Check sheet for the modelled part. Datum: model origin and axes. Units: mm. Face numbers are marked on the shaded views. A direction names the side the tool comes from. Coordinates: 2 decimals unless noted, no trailing zeros. Loops run counter-clockwise (first coordinate to the right, second up) from the corner with the lowest first, then second, coordinate; pieces in that order, holes last. Notation, with made-up numbers: (-26, -19.5) - (-22, -19.5) arc R14 ccw to (-22, 2.5) - close; hole circle Ø7 at (-33, 31.25). An arc over 180 degrees is marked (long way). Use a Markdown table: item, result. Add a question column.
1) Sectioned sample at D-D, the plane y = 11.5. Enter the section's corners in (x, z), then the cut area to 3 significant figures.
2) Sectioned sample at B-B, the plane x = 58. Enter the section's corners in (y, z), then the cut area to 3 significant figures.
3) Tool access check on the marked faces 4, 5, 6, 7 and 8. Record the directions out of +Z, -Z, +X, -X, +Y, -Y that give a thin tool (end or side, any length) a straight path to the whole face; none if there is none.
4) Thickness scan on line 1 (Y direction, x = 20, z = 9); line 2 (Z direction, x = 51.5, y = 18); line 3 (X direction, y = 25, z = -4.5). Record the ranges inside material, lowest first.
5) Go/stop test with flat-tipped pins: P1, Ø24, axis at x = 21.5, z = -36, coming from the -Y side; P2, Ø17.5, axis at x = 29.5, y = 60, coming from the -Z side; P3, Ø11, axis at x = 74, z = -43, coming from the -Y side; P4, Ø10, axis at y = 57.5, z = -71, coming from the -X side. Record where each tip stops, or that it passes through.
6) Sectioned sample at C-C, the plane x = 9. Enter the section's corners in (y, z).
7) Sectioned sample at A-A, the plane y = 40. Enter the section's corners in (x, z), then the cut area to 3 significant figures.
8) Draft check along Z on the marked faces 1, 2 and 3. Enter one of: pulls with the +Z half, pulls with the -Z half, needs draft (parallel to the pull), parting line crosses it, or undercut.
from build123d import *

# Parameters (mm, degrees)
BOSS_EXTRUDE1_DEPTH = 12
CUT_EXTRUDE1_REACH  = 115.772
SKETCH2_R           = 5
BOSS_EXTRUDE2_DEPTH = 10
SKETCH8_R           = 20
BOSS_EXTRUDE3_DEPTH = 30
CUT_EXTRUDE2_REACH  = 132.48
SKETCH9_R           = 12.5
BOSS_EXTRUDE4_DEPTH = 5


with BuildPart() as part:
    # Sketch1 → Boss-Extrude1 (new body)
    with BuildSketch(Plane.XY):
        with BuildLine():
            Line((20, 0), (80, 0))
            Line((80, 0), (80, 80))
            Line((80, 80), (20, 80))
            ThreePointArc((20, 80), (5.857864376, 74.142135624), (0, 60))
            Line((0, 60), (0, 20))
            ThreePointArc((0, 20), (5.857864376, 5.857864376), (20, 0))
        make_face()
    extrude(amount=BOSS_EXTRUDE1_DEPTH)

    # Sketch2 → Cut-Extrude1 (cut, up to next)
    with BuildSketch(Plane.XY.offset(12), mode=Mode.PRIVATE) as cut_extrude1_sk1:
        with Locations((20, 65)):
            Circle(SKETCH2_R)
    cut_extrude1_tool1 = extrude(cut_extrude1_sk1.sketch, amount=-CUT_EXTRUDE1_REACH, mode=Mode.PRIVATE) & part.part
    # Sketch2 → Cut-Extrude1 (cut, up to next)
    with BuildSketch(Plane.XY.offset(12), mode=Mode.PRIVATE) as cut_extrude1_sk2:
        with Locations((20, 15)):
            Circle(SKETCH2_R)
    cut_extrude1_tool2 = extrude(cut_extrude1_sk2.sketch, amount=-CUT_EXTRUDE1_REACH, mode=Mode.PRIVATE) & part.part
    add(cut_extrude1_tool1.solids().sort_by_distance((20, 65, 12))[0], mode=Mode.SUBTRACT)
    add(cut_extrude1_tool2.solids().sort_by_distance((20, 15, 12))[0], mode=Mode.SUBTRACT)

    # Sketch5 → Boss-Extrude2 (add)
    with BuildSketch(Plane(origin=(80, 0, 0), x_dir=(0, 0, -1), z_dir=(1, 0, 0))):
        with BuildLine():
            Line((10, 70), (65, 70))
            ThreePointArc((65, 70), (95, 40), (65, 10))
            Line((65, 10), (10, 10))
            ThreePointArc((10, 10), (2.928932188, 7.071067812), (0, 0))
            Line((0, 0), (0, 80))
            ThreePointArc((0, 80), (2.928932188, 72.928932188), (10, 70))
        make_face()
    extrude(amount=-BOSS_EXTRUDE2_DEPTH)

    # Sketch8 → Boss-Extrude3 (add)
    with BuildSketch(Plane.ZY.offset(-70)):
        with Locations(Location((-66.398885529, 40, 0), (0, 0, 180))):
            Circle(SKETCH8_R)
    extrude(amount=BOSS_EXTRUDE3_DEPTH)

    # Sketch9 → Cut-Extrude2 (cut, up to next)
    with BuildSketch(Plane.ZY.offset(-40), mode=Mode.PRIVATE) as cut_extrude2_sk1:
        with Locations((-66.398885529, 40)):
            Circle(SKETCH9_R)
    cut_extrude2_tool1 = extrude(cut_extrude2_sk1.sketch, amount=-CUT_EXTRUDE2_REACH, mode=Mode.PRIVATE) & part.part
    add(cut_extrude2_tool1.solids().sort_by_distance((40, 40, -66.398886))[0], mode=Mode.SUBTRACT)

    # Sketch16 → Boss-Extrude4 (add, symmetric)
    with BuildSketch(Plane(origin=(0, 40, 0), x_dir=(1, 0, 0), z_dir=(0, 1, 0))):
        with BuildLine():
            Line((40, 48.219297795), (70, 48.219297795))
            Line((70, 48.219297795), (70, 0))
            Line((70, 0), (0, 0))
            ThreePointArc((0, 0), (28.488651348, 17.067944239), (40, 48.219297795))
        make_face()
    extrude(amount=BOSS_EXTRUDE4_DEPTH, both=True)


solid = part.part
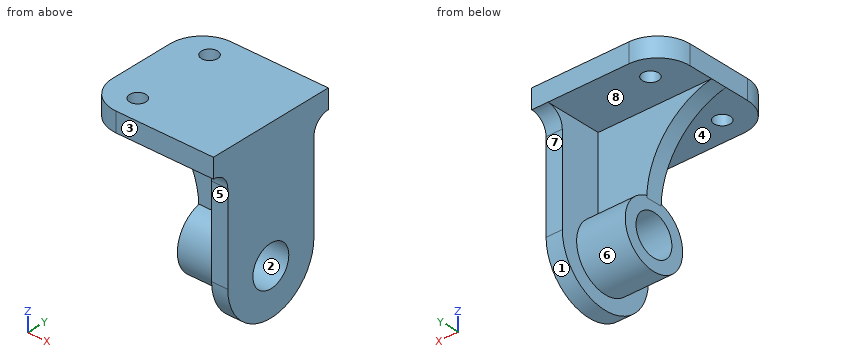
Solved:
| question | item | result |
|---|---|---|
| 1 | outline | (1.9, 0) - (16.43, 0) - (16.43, 12) - (1.9, 12) - close; (23.57, 0) - (70, 0) - (70, -74.37) - (80, -74.37) - (80, 12) - (23.57, 12) - close |
| 1 | area | 1,600 mm2 |
| 2 | outline | (0, 0) - (35, 0) - (35, -47.03) arc R20 ccw (long way) to (45, -47.03) - (45, 0) - (80, 0) - (80, 12) - (0, 12) - close; hole circle Ø25 at (40, -66.4) |
| 2 | area | 2,190 mm2 |
| 3 | face 4 | -X, -Y |
| 3 | face 5 | -Z, +X, -X, -Y |
| 3 | face 6 | -X |
| 3 | face 7 | -Z, +X, -X, +Y |
| 3 | face 8 | -X, +Y |
| 4 | line 1 | y = 0 to 10, 20 to 60, 70 to 80 |
| 4 | line 2 | z = 0 to 12 |
| 4 | line 3 | x = 70 to 80 |
| 5 | P1 | passes through |
| 5 | P2 | stops at z = 0 |
| 5 | P3 | stops at y = 10 |
| 5 | P4 | stops at x = 40 |
| 6 | outline | (3.3, 0) - (35, 0) - (35, -2.74) - (45, -2.74) - (45, 0) - (76.7, 0) - (76.7, 12) - (3.3, 12) - close |
| 7 | outline | (0, 0) arc R50 cw to (40, -48.22) - (40, -53.9) - (80, -53.9) - (80, 12) - (0, 12) - close; (40, -86.4) - (70, -86.4) - (70, -95) - (80, -95) - (80, -78.9) - (40, -78.9) - close |
| 7 | area | 3,990 mm2 |
| 8 | face 1 | pulls with the -Z half |
| 8 | face 2 | undercut |
| 8 | face 3 | needs draft |
